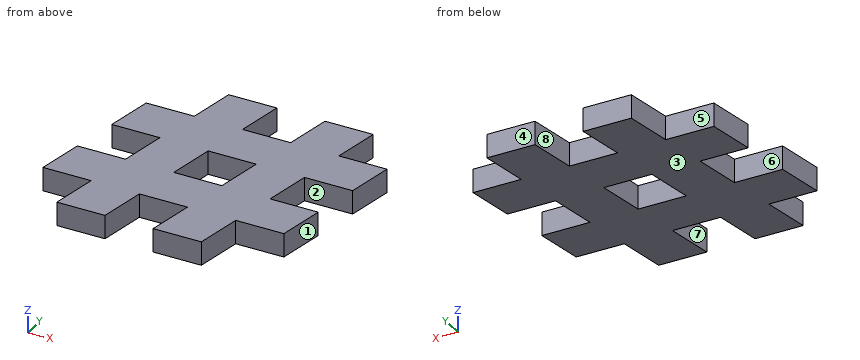
```python
from build123d import *

# Parameters (mm, degrees)
PAD_DEPTH = 3.175


with BuildPart() as part:
    # Sketch → Pad (new body)
    with BuildSketch(Plane.XY):
        Polygon((-14.424634, 9.514612), (-15.54309, 3.171537), (-9.102163, 3.171537), (-10.220618, -3.171537), (-16.661545, -3.171537), (-17.78, -9.514612), (-11.339073, -9.514612), (-12.457528, -15.857687), (-6.016601, -15.857687), (-4.898146, -9.514612), (1.542781, -9.514612), (0.424325, -15.857687), (6.865252, -15.857687), (7.983707, -9.514612), (14.424634, -9.514612), (15.54309, -3.171537), (9.102163, -3.171537), (10.220618, 3.171537), (16.661545, 3.171537), (17.78, 9.514612), (11.339073, 9.514612), (12.457528, 15.857687), (6.016601, 15.857687), (4.898146, 9.514612), (-1.542781, 9.514612), (-0.424325, 15.857687), (-6.865252, 15.857687), (-7.983707, 9.514612), align=None)
        Polygon((-2.661236, 3.171537), (-3.779691, -3.171537), (2.661236, -3.171537), (3.779691, 3.171537), align=None, mode=Mode.SUBTRACT)
    extrude(amount=PAD_DEPTH)


solid = part.part
```
Here's how the part is built. I have some questions about the finished solid (model axes, mm). Face numbers are marked on the shaded views. A direction names the side the tool comes from. Round coordinates to 2 decimals unless told otherwise and drop trailing zeros. Loops run counter-clockwise (first coordinate to the right, second up) from the corner with the lowest first, then second, coordinate; pieces in that order, holes last. Notation, with made-up numbers: (18, 62) -> (37, 62) arc R30 ccw to (37, 95) -> close; hole circle Ø6 at (-21.5, 83.25). An arc over 180 degrees is marked (long way). Answer as CSV lines item,"result".
1. Thinking about a two-plate mould opening in Y: for the marked faces 1, 2, 3 and 4, which applies, released by +Y, released by -Y, zero draft, split by the parting line, or undercut?
Final values:
face 1,"released by -Y"
face 2,"undercut"
face 3,"zero draft"
face 4,"released by +Y"
2. If we section it at D-D on y = -7.5: Please give me the cut outline in (x, z) (3 decimals).
Final values:
outline,"(-17.425, 0) -> (14.78, 0) -> (14.78, 3.175) -> (-17.425, 3.175) -> close"
3. If we section it at C-C on y = 13: Please give me the cut outline in (x, z) (3 decimals), plus the area to 3 significant figures.
Final values:
outline,"(-7.369, 0) -> (-0.928, 0) -> (-0.928, 3.175) -> (-7.369, 3.175) -> close; (5.513, 0) -> (11.954, 0) -> (11.954, 3.175) -> (5.513, 3.175) -> close"
area,"40.9 mm^2"
4. For pin 1 (1 mm diameter, centred on x = 14, y = 1.5, fed in from +Z); pin 2 (1 mm diameter, centred on x = -12.5, z = 1.5, fed in from +Y); pin 3 (1.6 mm diameter, centred on x = -14, z = 1.5, fed in from -Y), each with a flat end and sliding along its axis, tell me the tip position at first contact or that it passes through.
Final values:
pin 1,"passes through"
pin 2,"stops at y = 9.51"
pin 3,"stops at y = -9.51"
5. Which directions (+Z, -Z, +X, -X, +Y, -Y) give clear straight access to the entire face, cutting with the end or side of a thin tool? Please do the marked faces 5, 6, 7 and 8.
Final values:
face 5,"+Z, -Z, -X, +Y"
face 6,"+Z, -Z, -X"
face 7,"+Z, -Z"
face 8,"+Z, -Z, +Y"
6. If we section it at B-B on x = 15: Please give me the cut outline in (y, z) (3 decimals).
Final values:
outline,"(-6.252, 0) -> (-3.172, 0) -> (-3.172, 3.175) -> (-6.252, 3.175) -> close; (3.172, 0) -> (9.515, 0) -> (9.515, 3.175) -> (3.172, 3.175) -> close"
7. If I drill on L1, parallel to Y at x = -13, z = 1; L2, parallel to Y at x = 2.5, z = 2.2; L3, parallel to X at y = 14.5, z = 1, over which ranges is the centre line in solid material (lowest first)?
Final values:
L1,"y = -9.51 to -3.17, 3.17 to 9.51"
L2,"y = -15.86 to -3.17, 3.17 to 9.51"
L3,"x = -7.1 to -0.66, 5.78 to 12.22"
